Check sheet for the modelled part. Datum: model origin and axes. Units: mm. A direction names the side the tool comes from. Give positions to 0.01 mm unless a question says otherwise; leave off trailing zeros. Answer as a JSON object with one key per item and string values.
from build123d import *

# Parameters (mm, degrees)
DODANIE_WYCI_GNI_CIE2_DEPTH = 1
WYTNIJ_WYCI_GNI_CIE1_DEPTH  = 32.093249288
SZKIC4_W                    = 30
SZKIC4_H                    = 28
DODANIE_WYCI_GNI_CIE3_DEPTH = 1.5
SZKIC3_W                    = 30
SZKIC3_H                    = 1
DODANIE_WYCI_GNI_CIE4_DEPTH = 10
ZAOKR_GLENIE1_R             = 0.3
ZAOKR_GLENIE2_R             = 0.5
ZAOKR_GLENIE3_R             = 0.2


with BuildPart() as part:
    # Szkic1 → Dodanie-wyciągnięcie2 (new body)
    with BuildSketch(Plane(origin=(0, 0, 0), x_dir=(1, 0, 0), z_dir=(0, 1, 0))):
        with BuildLine():
            ThreePointArc((-14.974873734, 18.474873734), (-15.24129537, 19.814265747), (-16, 20.949747468))
            Line((-16, 20.949747468), (-20.949747468, 16))
            ThreePointArc((-20.949747468, 16), (-18.474873734, 14.974873734), (-16, 16))
            ThreePointArc((-16, 16), (-15.24129537, 17.135481721), (-14.974873734, 18.474873734))
        make_face()
        with BuildLine():
            Line((-20.949747468, 16), (-16, 20.949747468))
            ThreePointArc((-16, 20.949747468), (-20.949747468, 20.949747468), (-20.949747468, 16))
        make_face()
        with BuildLine():
            Line((-11.050252532, 16), (-16, 20.949747468))
            ThreePointArc((-16, 20.949747468), (-15.24129537, 19.814265747), (-14.974873734, 18.474873734))
            ThreePointArc((-14.974873734, 18.474873734), (-15.24129537, 17.135481721), (-16, 16))
            Line((-16, 16), (-11.050252532, 16))
        make_face()
        Polygon((16, -11.050252532), (-11.050252532, 16), (-16, 16), (-16, 11.050252532), (11.050252532, -16), (16, -16), align=None)
        with BuildLine():
            ThreePointArc((-16, 16), (-18.474873734, 14.974873734), (-20.949747468, 16))
            Line((-20.949747468, 16), (-16, 11.050252532))
            Line((-16, 11.050252532), (-16, 16))
        make_face()
        Polygon((11.050252532, -16), (-16, 11.050252532), (-16, -16), align=None)
        Polygon((16, 16), (-11.050252532, 16), (16, -11.050252532), align=None)
        with BuildLine():
            Line((20.949747468, -16), (16, -11.050252532))
            Line((16, -11.050252532), (16, -16))
            ThreePointArc((16, -16), (18.474873734, -14.974873734), (20.949747468, -16))
        make_face()
        with BuildLine():
            ThreePointArc((21.974873734, -18.474873734), (21.708452098, -17.135481721), (20.949747468, -16))
            Line((20.949747468, -16), (16, -20.949747468))
            ThreePointArc((16, -20.949747468), (19.814265747, -21.708452098), (21.974873734, -18.474873734))
        make_face()
        with BuildLine():
            Line((16, -20.949747468), (20.949747468, -16))
            ThreePointArc((20.949747468, -16), (18.474873734, -14.974873734), (16, -16))
            ThreePointArc((16, -16), (14.974873734, -18.474873734), (16, -20.949747468))
        make_face()
        with BuildLine():
            ThreePointArc((16, -20.949747468), (14.974873734, -18.474873734), (16, -16))
            Line((16, -16), (11.050252532, -16))
            Line((11.050252532, -16), (16, -20.949747468))
        make_face()
    extrude(amount=DODANIE_WYCI_GNI_CIE2_DEPTH)

    # Szkic2 → Wytnij-wyciągnięcie1 (cut, through all)
    with BuildSketch(Plane(origin=(0, 1, 0), x_dir=(1, 0, 0), z_dir=(0, 1, 0))):
        with BuildLine():
            Line((-17.414213562, 19.535533906), (-14.939339828, 17.060660172))
            ThreePointArc((-14.939339828, 17.060660172), (-14.939339828, 14.939339828), (-17.060660172, 14.939339828))
            Line((-17.060660172, 14.939339828), (-19.535533906, 17.414213562))
            ThreePointArc((-19.535533906, 17.414213562), (-19.535533906, 19.535533906), (-17.414213562, 19.535533906))
        make_face()
        with BuildLine():
            Line((19.535533906, -17.414213562), (17.060660172, -14.939339828))
            ThreePointArc((17.060660172, -14.939339828), (14.939339828, -14.939339828), (14.939339828, -17.060660172))
            Line((14.939339828, -17.060660172), (17.414213562, -19.535533906))
            ThreePointArc((17.414213562, -19.535533906), (19.535533906, -19.535533906), (19.535533906, -17.414213562))
        make_face()
    extrude(amount=-WYTNIJ_WYCI_GNI_CIE1_DEPTH, mode=Mode.SUBTRACT)

    # Szkic4 → Dodanie-wyciągnięcie3 (add)
    with BuildSketch(Plane(origin=(0, 1, 0), x_dir=(1, 0, 0), z_dir=(0, 1, 0))):
        Rectangle(SZKIC4_W, SZKIC4_H)
    extrude(amount=DODANIE_WYCI_GNI_CIE3_DEPTH)

    # Szkic3 → Dodanie-wyciągnięcie4 (add)
    with BuildSketch(Plane(origin=(0, 1, 0), x_dir=(1, 0, 0), z_dir=(0, 1, 0))):
        with Locations((0, 13.5)):
            Rectangle(SZKIC3_W, SZKIC3_H)
        with Locations((0, 4.5)):
            Rectangle(SZKIC3_W, SZKIC3_H)
        with Locations((0, -4.5)):
            Rectangle(SZKIC3_W, SZKIC3_H)
        with Locations((0, -11.25)):
            Rectangle(SZKIC3_W, SZKIC3_H)
        with Locations((0, -13.5)):
            Rectangle(SZKIC3_W, SZKIC3_H)
        with Locations((0, 11.25)):
            Rectangle(SZKIC3_W, SZKIC3_H)
        with Locations((0, 9)):
            Rectangle(SZKIC3_W, SZKIC3_H)
        with Locations((0, 6.75)):
            Rectangle(SZKIC3_W, SZKIC3_H)
        with Locations((0, 2.25)):
            Rectangle(SZKIC3_W, SZKIC3_H)
        Rectangle(SZKIC3_W, SZKIC3_H)
        with Locations((0, -2.25)):
            Rectangle(SZKIC3_W, SZKIC3_H)
        with Locations((0, -6.75)):
            Rectangle(SZKIC3_W, SZKIC3_H)
        with Locations((0, -9)):
            Rectangle(SZKIC3_W, SZKIC3_H)
    extrude(amount=DODANIE_WYCI_GNI_CIE4_DEPTH)

    # Zaokrąglenie1
    zaokr_glenie1_edges = [part.edges().sort_by_distance(p)[0] for p in [
        (0, 11, -5),
        (0, 11, -4),
        (0, 11, 4),
        (0, 11, 5),
        (0, 11, 10.75),
        (0, 11, 11.75),
        (0, 11, 13),
        (0, 11, 14),
        (0, 11, -11.75),
        (0, 11, -10.75),
        (0, 11, -9.5),
        (0, 11, -8.5),
        (0, 11, -7.25),
        (0, 11, -6.25),
        (0, 11, -2.75),
        (0, 11, -1.75),
        (0, 11, -0.5),
        (0, 11, 0.5),
        (0, 11, 1.75),
        (0, 11, 2.75),
        (0, 11, 6.25),
        (0, 11, 7.25),
        (0, 11, 8.5),
        (0, 11, 9.5),
        (0, 11, -14),
        (0, 11, -13),
    ]]
    fillet(zaokr_glenie1_edges, radius=ZAOKR_GLENIE1_R)

    # Zaokrąglenie2
    zaokr_glenie2_edges = [part.edges().sort_by_distance(p)[0] for p in [
        (0, 2.5, -4),
        (0, 2.5, -5),
        (0, 2.5, 5),
        (0, 2.5, 4),
        (0, 2.5, 11.75),
        (0, 2.5, 10.75),
        (0, 2.5, 13),
        (0, 2.5, -10.75),
        (0, 2.5, -11.75),
        (0, 2.5, -8.5),
        (0, 2.5, -9.5),
        (0, 2.5, -6.25),
        (0, 2.5, -7.25),
        (0, 2.5, -1.75),
        (0, 2.5, -2.75),
        (0, 2.5, 0.5),
        (0, 2.5, -0.5),
        (0, 2.5, 2.75),
        (0, 2.5, 1.75),
        (0, 2.5, 7.25),
        (0, 2.5, 6.25),
        (0, 2.5, 9.5),
        (0, 2.5, 8.5),
        (0, 2.5, -13),
    ]]
    fillet(zaokr_glenie2_edges, radius=ZAOKR_GLENIE2_R)

    # Zaokrąglenie3
    zaokr_glenie3_edges = [part.edges().sort_by_distance(p)[0] for p in [
        (-15, 1, 0),
        (0, 1, 14),
        (15, 1, 0),
        (0, 1, -14),
    ]]
    fillet(zaokr_glenie3_edges, radius=ZAOKR_GLENIE3_R)


solid = part.part
1. Scan lines: L1, parallel to X at y = 7.5, z = -7; L2, parallel to Y at x = 7, z = 2; L3, parallel to Y at x = -8.5, z = 15. Record each from-to range of solid material in increasing order. Write a range as [from, to].
Determined:
{"L1": "[-15, 15]", "L2": "[0, 11]", "L3": "[0, 1]"}
2. Mould release check, pull along X, two halves, no side actions. Record for faces 4 (the face through (16, 0.5, -2.3)), 5 (the face through (0, 7, -1.75)), 6 (the face through (18.315, 0.507, 16.194)): released by +X, released by -X, zero draft, split by the parting line, or undercut.
Determined:
{"face 4": "released by +X", "face 5": "zero draft", "face 6": "undercut"}
3. Go/stop test with flat-tipped pins: P1, Ø4, axis at x = 6, y = 6, coming from the -Z side; P2, Ø1.5, axis at x = -2.5, y = 3, coming from the +Z side; P3, Ø5, axis at x = 13.5, z = 8.5, coming from the +Y side; P4, Ø1.1, axis at x = -9, y = 0.5, coming from the +Z side. Record where each tip stops, or that it passes through.
Determined:
{"P1": "z = -14", "P2": "z = 14", "P3": "y = 11", "P4": "z = 16"}
4. Access from +Z, -Z, +X, -X, +Y, -Y to the whole of each face (thin tool, end or side, straight path). Record for faces 1 (the face through (-16.194, 0.507, -18.315)), 2 (the face through (0, 7, -6.25)), 3 (the face through (-2.7, 0.5, 16)).
Determined:
{"face 1": "+Y, -Y", "face 2": "+X, -X, +Y", "face 3": "+Z, -X, +Y, -Y"}
5. Sectioned sample at A-A, the plane y = 4.5. State how many separate pieces and enclosed holes the cut face has, plus the area to 3 significant figures.
Determined:
{"separate pieces": "13", "enclosed holes": "0", "area": "390 mm^2"}
